Part model, mm, in its own coordinate system. Face numbers are marked on the shaded views. A direction names the side the tool comes from. Coordinates: 2 decimals unless noted, no trailing zeros. Loops run counter-clockwise (first coordinate to the right, second up) from the corner with the lowest first, then second, coordinate; pieces in that order, holes last. Notation, with made-up numbers: (82, 46.5) - (123, 46.5) arc R12 cw to (123, 62.5) - close; hole circle Ø1 at (70, 48.25). An arc over 180 degrees is marked (long way). Use a Markdown table: item, result. Add a question column.
1. Band-saw the part on B-B, the plane z = 1.5. Count the separate pieces of the cut face and the enclosed holes in it, plus the area to 3 significant figures.
2. Drop flat-ended pins along their axis: pin 1 (6.5 mm diameter, centred on x = 10.67, y = -52.6, fed in from +Z); pin 2 (1.5 mm diameter, centred on x = -16.5, z = 8.5, fed in from -Y); pin 3 (4 mm diameter, centred on x = 2, y = -56, fed in from -Z); pin 4 (3.5 mm diameter, centred on x = -41.89, y = -66.54, fed in from +Z). Give the stop position or say it passes through.
3. Wall check: probe 1 along Y at (x, z) = (-53, 4.5); probe 2 along Z at (x, y) = (-11, -62); probe 3 along Y at (x, z) = (-21, 0.75). Give the ranges that are in metal, low to high. Write a range as [from, to].
4. 3-axis set-ups, long thin cutter, end or side, ignore diameter. For the marked faces 5, 6 and 7: which of +Z, -Z, +X, -X, +Y, -Y reach the whole face in a straight line?
5. Band-saw the part on A-A, the plane z = 16. Give the cut face in (x, y).
6. Pull direction X, two halves, no side cores. Call the marked faces 1, 2, 3 and 4: pulls with the +X half, pulls with the -X half, needs draft (parallel to the pull), parting line crosses it, or undercut.
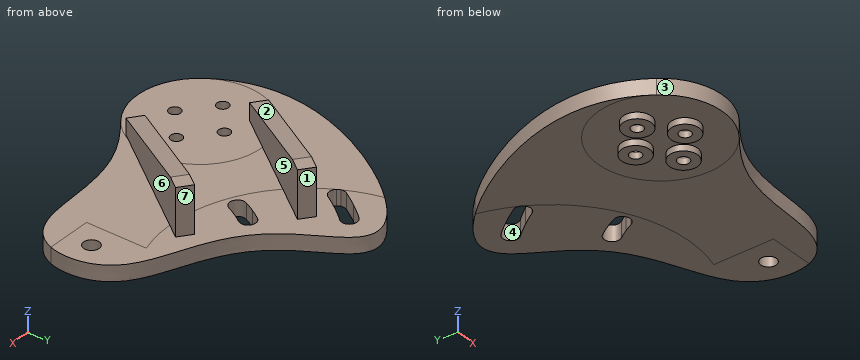
Autodesk Inventor part; units mm, degrees
ref_plane "YZ Plane" through (0, 0, 0) normal (1, 0, 0) x (0, 1, 0)
ref_plane "XZ Plane" through (0, 0, 0) normal (0, 1, 0) x (-1, 0, 0)
ref_plane "XY Plane" through (0, 0, 0) normal (0, 0, 1) x (1, 0, 0)
ref_plane "Work Plane1" through (0, 0, 0) normal (0, 0, 1) x (1, 0, 0)
sketch "Sketch1" plane through (0, 0, 0) normal (0, 0, 1) x (1, 0, 0)
  circle A0 centre (-25.0838, -31.7051) radius 2.5
  circle A1 centre (-43.012, -13.2629) radius 2.5
  circle A2 centre (-44.8914, 13.7567) radius 2.5
  circle A3 centre (-28.0838, 36.7109) radius 2.5
  circle A4 centre (0.8935, 43.7288) radius 2.5
  circle A5 centre (29.5533, 30.4373) radius 2.5
  circle A6 centre (43.6662, -0.0951) radius 2.5
  circle A7 centre (47.6662, -52.5951) radius 2.5
  circle A8 centre (10.6662, -52.5951) radius 2.5
  circle A9 centre (-6.8338, -0.0951) radius 8.75
  line L0 (56.6662, -60.0951) -> (51.1662, -0.0951)
  spline S0 degree 4 poles (51.1662, -0.0951) (50.0319, 24.6801) (26.25, 55.8136) (-25.1104, 60.0951) (-56.6662, 18.5311) (-54.7055, -22.2338) (-29.645, -43.1708) (-8.3823, -44.3792) (3.1662, -40.8213) knots 0 0 0 0 0 0.330099 0.457579 0.582312 0.704438 0.895347 0.895347 0.895347 0.895347 0.895347
  line L1 (3.1662, -40.8213) -> (3.1662, -60.0951)
  line L2 (3.1662, -60.0951) -> (56.6662, -60.0951)
  circle A10 centre (-6.8338, -0.0951) radius 80 construction
  circle A11 centre (-51.3856, -66.5416) radius 20
  spline S1 degree 4 poles (-67.6748, -78.146) (-80.1343, -60.6563) (-73.4442, -28.8039) (-34.6199, 23.5084) (-28.149, -22.306) (-1.1527, -34.0954) (21.6131, -40.077) (20.0804, -79.4594) (-16.1771, -65.3424) (-30.503, -75.865) (-39.3686, -82.5289) knots 0 0 0 0 0 0.227581 0.363335 0.480166 0.59047 0.703016 0.817261 1 1 1 1 1
  line L3 (10.6662, -52.5951) -> (-43.012, -13.2629) construction
  line L4 (-25.0838, -31.7051) -> (10.6662, -52.5951) construction
  line L5 (10.6662, -52.5951) -> (-42.0733, -6.3735) construction
  line L6 (10.6662, -52.5951) -> (-49.6403, -16.0265) construction
  arc A12 (-37.4996, -10.382) -> (-40.9954, -14.7405) centre (10.6662, -52.5951) ccw
  arc A13 (-40.9954, -14.7405) -> (-44.098, -19.3872) centre (10.6662, -52.5951) ccw
  arc A14 (-41.2598, -7.0865) -> (-45.0286, -11.7853) centre (10.6662, -52.5951) ccw
  arc A15 (-45.0286, -11.7853) -> (-48.3734, -16.7947) centre (10.6662, -52.5951) ccw
  arc A16 (-37.4996, -10.382) -> (-41.2598, -7.0865) centre (-39.3797, -8.7342) ccw
  arc A17 (-48.3734, -16.7947) -> (-44.098, -19.3872) centre (-46.2357, -18.0909) ccw
  line L7 (10.6662, -52.5951) -> (-30.2455, -33.2568) construction
  line L8 (10.6662, -52.5951) -> (-26.0132, -26.6253) construction
  arc A18 (-21.0867, -30.1134) -> (-24.5082, -35.9687) centre (10.6662, -52.5951) ccw
  arc A19 (-25.1674, -27.2241) -> (-29.0287, -33.832) centre (10.6662, -52.5951) ccw
  arc A20 (-21.0867, -30.1134) -> (-25.1674, -27.2241) centre (-23.1271, -28.6687) ccw
  arc A21 (-29.0287, -33.832) -> (-24.5082, -35.9687) centre (-26.7685, -34.9004) ccw
  point P0 (0, 0)
  point P1 (-60.5912, -17.8314)
  point P2 (-36.7792, -0.096)
  point P3 (-23.1279, -18.1974)
  point P4 (0.0342, -33.7731)
  point P5 (16.7837, -45.8922)
  point P6 (15.1081, -64.5601)
  point P7 (-10.6842, -70.5676)
  point P8 (-45.0286, -11.7853)
  point P9 (-21.0867, -30.1134)
  dimension "d0" = 160
  dimension "d1" = 40
  dimension "d2" = 5
  dimension "d3" = 5
  dimension "d4" = 2.5
  dimension "d5" = 5
  dimension "d6" = 5
extrude "Extrusion1" add sketch "Sketch1" along normal blind 5 contours A15 A17 S0 S1 L2 L1 A13 A12 A16 A14 | A11 | A17 S0 L1 L2 S1 A11
sketch "Sketch2" plane through (0, 0, 0) normal (0, 0, -1) x (-1, 0, 0)
  arc A0 (39.3686, -82.5289) -> (67.6748, -78.146) centre (51.3856, -66.5416) ccw
  circle A1 centre (51.3856, -66.5416) radius 8 construction
  circle A2 centre (51.3856, -66.5416) radius 9.5 construction
  point P0 (0, 0)
  point P1 (60.8856, -66.5416)
  point P2 (41.8856, -66.5416)
  point P3 (51.3856, -74.5416)
  point P4 (51.3856, -58.5416)
  dimension "d9" = 16
  dimension "d10" = 19
hole "Hole1" at (-60.8856, -66.5416, 0) at (-41.8856, -66.5416, 0) at (-51.3856, -74.5416, 0) at (-51.3856, -58.5416, 0) direction (0, 0, 1) diameter 3.7 end through all
sketch "Sketch3" plane through (0, 0, 0) normal (0, 0, -1) x (-1, 0, 0)
  circle A0 centre (51.3856, -58.5416) radius 1.85
  circle A1 centre (51.3856, -74.5416) radius 1.85
  circle A2 centre (41.8856, -66.5416) radius 1.85
  circle A3 centre (60.8856, -66.5416) radius 1.85
  arc A4 (39.3686, -82.5289) -> (67.6748, -78.146) centre (51.3856, -66.5416) ccw
  arc A5 (44.098, -19.3872) -> (48.3734, -16.7947) centre (46.2357, -18.0909) ccw
  arc A6 (44.098, -19.3872) -> (37.4996, -10.382) centre (-10.6662, -52.5951) ccw
  arc A7 (41.2598, -7.0865) -> (37.4996, -10.382) centre (39.3797, -8.7342) ccw
  arc A8 (48.3734, -16.7947) -> (41.2598, -7.0865) centre (-10.6662, -52.5951) ccw
  arc A9 (25.1674, -27.2241) -> (21.0867, -30.1134) centre (23.1271, -28.6687) ccw
  arc A10 (29.0287, -33.832) -> (25.1674, -27.2241) centre (-10.6662, -52.5951) ccw
  arc A11 (24.5082, -35.9687) -> (29.0287, -33.832) centre (26.7685, -34.9004) ccw
  arc A12 (24.5082, -35.9687) -> (21.0867, -30.1134) centre (-10.6662, -52.5951) ccw
  circle A13 centre (-10.6662, -52.5951) radius 2.5
  circle A14 centre (60.8856, -66.5416) radius 4.5
  circle A15 centre (51.3856, -74.5416) radius 4.5
  circle A16 centre (41.8856, -66.5416) radius 4.5
  circle A17 centre (51.3856, -58.5416) radius 4.5
  point P0 (0, 0)
  dimension "d18" = 9
  dimension "d19" = 9
  dimension "d20" = 9
  dimension "d21" = 9
extrude "Extrusion2" add sketch "Sketch3" along normal blind 2 contours A14 | A15 | A16 | A17
sketch "Sketch4" plane through (0, 0, 5) normal (0, 0, 1) x (1, 0, 0)
  circle A0 centre (-51.3856, -58.5416) radius 1.85
  circle A1 centre (-51.3856, -74.5416) radius 1.85
  circle A2 centre (-41.8856, -66.5416) radius 1.85
  circle A3 centre (-60.8856, -66.5416) radius 1.85
  arc A4 (-67.6748, -78.146) -> (-39.3686, -82.5289) centre (-51.3856, -66.5416) ccw
  arc A5 (-48.3734, -16.7947) -> (-44.098, -19.3872) centre (-46.2357, -18.0909) ccw
  arc A6 (-41.2598, -7.0865) -> (-48.3734, -16.7947) centre (10.6662, -52.5951) ccw
  arc A7 (-37.4996, -10.382) -> (-41.2598, -7.0865) centre (-39.3797, -8.7342) ccw
  arc A8 (-37.4996, -10.382) -> (-44.098, -19.3872) centre (10.6662, -52.5951) ccw
  arc A9 (-21.0867, -30.1134) -> (-25.1674, -27.2241) centre (-23.1271, -28.6687) ccw
  arc A10 (-21.0867, -30.1134) -> (-24.5082, -35.9687) centre (10.6662, -52.5951) ccw
  arc A11 (-29.0287, -33.832) -> (-24.5082, -35.9687) centre (-26.7685, -34.9004) ccw
  arc A12 (-25.1674, -27.2241) -> (-29.0287, -33.832) centre (10.6662, -52.5951) ccw
  circle A13 centre (10.6662, -52.5951) radius 2.5
  line L0 (-35.0492, -15.9402) -> (-63.5128, -53.8187)
  line L1 (-63.5128, -53.8187) -> (-59.5155, -56.8224)
  line L2 (-59.5155, -56.8224) -> (-31.0519, -18.9439)
  line L3 (-31.0519, -18.9439) -> (-35.0492, -15.9402)
  line L4 (-9.4669, -35.1638) -> (-38.9594, -74.4116)
  line L5 (-38.9594, -74.4116) -> (-34.9622, -77.4153)
  line L6 (-34.9622, -77.4153) -> (-5.4697, -38.1675)
  line L7 (-5.4697, -38.1675) -> (-9.4669, -35.1638)
  point P0 (0, 0)
  dimension "d24" = 5
  dimension "d25" = 5
  dimension "d26" = 27
extrude "Extrusion3" add sketch "Sketch4" along normal blind 15 contours L3 L2 L1 L0 | L7 L6 L5 L4
sketch "Sketch5" plane through (-63.5128, -53.8187, 5) normal (-0.7994, 0.6007, 0) x (0, 0, 1)
  line L0 (0, 0) -> (0, 47.381)
  line L1 (0, 0) -> (15, 0)
  line L2 (15, 47.381) -> (15, 0)
  line L3 (0, 47.381) -> (15, 47.381)
  line L4 (15, 0) -> (15, 47.381)
  line L5 (15, 42.381) -> (5, -1.85)
  line L6 (5, -1.85) -> (0, -1.85)
  line L7 (0, -1.85) -> (0, 0)
  line L8 (15, 42.381) -> (15, -1.85)
  line L9 (15, -1.85) -> (5, -1.85)
  point P0 (-5, 81.1797)
  dimension "d29" = 5
  dimension "d30" = 5
extrude "Extrusion4" cut sketch "Sketch5" against normal blind 41.9875 contours L5 L2 L1 | L1 L8 L9 L5
properties part number "Soporte motor 2"
Geometry check:
| question | item | result |
|---|---|---|
| 1 | separate pieces | 1 |
| 1 | enclosed holes | 7 |
| 1 | area | 4,780 mm^2 |
| 2 | pin 1 | stops at z = 5 |
| 2 | pin 2 | stops at y = -53.84 |
| 2 | pin 3 | stops at z = 0 |
| 2 | pin 4 | passes through |
| 3 | probe 1 | y = [-86.48, -75.45], [-73.64, -59.45], [-57.64, -8.11] |
| 3 | probe 2 | z = [0, 5] |
| 3 | probe 3 | y = [-72.43, -29.98], [-27.35, -20.78] |
| 4 | face 5 | +Z |
| 4 | face 6 | +Z, +X, -Y |
| 4 | face 7 | +Z, +X, +Y |
| 5 | outline | (-48.68, -34.08) - (-44.68, -37.09) - (-31.05, -18.94) - (-35.05, -15.94) - close; (-23.1, -53.31) - (-19.1, -56.31) - (-5.47, -38.17) - (-9.47, -35.16) - close |
| 6 | face 1 | pulls with the +X half |
| 6 | face 2 | pulls with the -X half |
| 6 | face 3 | parting line crosses it |
| 6 | face 4 | undercut |
